CAD build for the part. Positions are in the model's coordinates, mm. Face numbers are marked on the shaded views. Round coordinates to 2 decimals unless told otherwise and drop trailing zeros. Order: outer loops, then holes, each group sorted by start corner. A loop starts at its lowest first (then second) coordinate and runs counter-clockwise, first axis right, second up. Notation, with made-up numbers: (52.5, 54) -> (83.5, 54) arc R17 ccw to (83.5, 66) -> close; hole circle Ø9 at (32, -39). An arc over 180 degrees is marked (long way). Return JSON: item names as keys, results as strings. Group by question number.
Q1. Flat gauge pins, fed straight in: pin 1 (3 mm diameter, centred on y = 1208, z = 845, fed in from +X); pin 2 (3 mm diameter, centred on x = 1200, z = 6, fed in from +Y); pin 3 (5 mm diameter, centred on x = 524.5, z = 487, fed in from -Y). Where does each tip first touch, or does it go through?
Q2. Mould opens along Z. For the marked faces 1, 2 and 3 say: +Z half, -Z half, draft (parallel to the pull), parting line (faces both ways), or undercut.
Q3. Cut at B-B (z = 315). Write the cut outline in (x, y), then the cut area to 3 significant figures.
Q4. Cut at A-A (y = 234). Write the cut outline in (x, z).
Q5. Probe line 1 along Z through (x, y) = (1775, 1221); line 2 along Y through (x, z) = (1104, 408.5); line 3 along X through (y, z) = (845.5, 64). List the from-to ranges inside material, lowest first.
from build123d import *

# Parameters (mm, degrees)
CROQUIS2_W                = 76.2
CROQUIS2_H                = 76.2
SALIENTE_EXTRUIR1_DEPTH   = 900
SALIENTE_EXTRUIR1_2_DEPTH = 900
SALIENTE_EXTRUIR1_3_DEPTH = 900
SALIENTE_EXTRUIR1_4_DEPTH = 900
CROQUIS3_W                = 1852.4
CROQUIS3_H                = 852.4
SALIENTE_EXTRUIR2_DEPTH   = 210
CROQUIS4_W                = 832.4
CROQUIS4_H                = 150
CORTAR_EXTRUIR1_DEPTH     = 1852.4
CROQUIS5_W                = 110
CROQUIS5_H                = 10
SALIENTE_EXTRUIR3_DEPTH   = 220
CROQUIS6_R                = 12.7
SALIENTE_EXTRUIR4_DEPTH   = 40
SALIENTE_EXTRUIR5_START   = -40
CROQUIS7_R                = 12.7
SALIENTE_EXTRUIR5_DEPTH   = 40
CROQUIS8_R                = 44.45
SALIENTE_EXTRUIR6_DEPTH   = 772.4


with BuildPart() as part:
    # Croquis2 → Saliente-Extruir1 (new body)
    with BuildSketch(Plane(origin=(0, 0, 0), x_dir=(1, 0, 0), z_dir=(0, 1, 0))):
        with Locations((38.1, -38.1)):
            Rectangle(CROQUIS2_W, CROQUIS2_H)
    extrude(amount=SALIENTE_EXTRUIR1_DEPTH)



with BuildPart() as body_2:
    # Croquis2 → Saliente-Extruir1 2 (new body)
    with BuildSketch(Plane(origin=(0, 0, 0), x_dir=(1, 0, 0), z_dir=(0, 1, 0))):
        with Locations((1814.3, -38.1)):
            Rectangle(CROQUIS2_W, CROQUIS2_H)
    extrude(amount=SALIENTE_EXTRUIR1_2_DEPTH)


with BuildPart() as body_3:
    # Croquis2 → Saliente-Extruir1 3 (new body)
    with BuildSketch(Plane(origin=(0, 0, 0), x_dir=(1, 0, 0), z_dir=(0, 1, 0))):
        with Locations((1814.3, -814.3)):
            Rectangle(CROQUIS2_W, CROQUIS2_H)
    extrude(amount=SALIENTE_EXTRUIR1_3_DEPTH)


with BuildPart() as body_4:
    # Croquis2 → Saliente-Extruir1 4 (new body)
    with BuildSketch(Plane(origin=(0, 0, 0), x_dir=(1, 0, 0), z_dir=(0, 1, 0))):
        with Locations((38.1, -814.3)):
            Rectangle(CROQUIS2_W, CROQUIS2_H)
    extrude(amount=SALIENTE_EXTRUIR1_4_DEPTH)


with BuildPart() as part_1:
    add(part.part)

    add(body_2.part)  # Saliente-Extruir2 merges body 2

    add(body_3.part)  # Saliente-Extruir2 merges body 3

    add(body_4.part)  # Saliente-Extruir2 merges body 4
    # Croquis3 → Saliente-Extruir2 (add)
    with BuildSketch(Plane(origin=(0, 900, 0), x_dir=(1, 0, 0), z_dir=(0, 1, 0))):
        with Locations((926.2, -426.2)):
            Rectangle(CROQUIS3_W, CROQUIS3_H)
    extrude(amount=SALIENTE_EXTRUIR2_DEPTH)

    # Croquis4 → Cortar-Extruir1 (cut)
    with BuildSketch(Plane.ZY):
        with Locations((426.2, 1035)):
            Rectangle(CROQUIS4_W, CROQUIS4_H)
    extrude(amount=-CORTAR_EXTRUIR1_DEPTH, mode=Mode.SUBTRACT)

    # Croquis5 → Saliente-Extruir3 (add)
    with BuildSketch(Plane(origin=(0, 1110, 0), x_dir=(1, 0, 0), z_dir=(0, 1, 0))):
        with Locations((1747.4, -5)):
            Rectangle(CROQUIS5_W, CROQUIS5_H)
        with Locations((1747.4, -847.4)):
            Rectangle(CROQUIS5_W, CROQUIS5_H)
    extrude(amount=SALIENTE_EXTRUIR3_DEPTH)

    # Croquis6 → Saliente-Extruir4 (add)
    with BuildSketch(Plane.XY.offset(852.4)):
        with Locations((1747.4, 1280)):
            Circle(CROQUIS6_R)
    extrude(amount=-SALIENTE_EXTRUIR4_DEPTH)

    # Croquis7 → Saliente-Extruir5 (add)
    with BuildSketch(Plane(origin=(0, 0, 0), x_dir=(-1, 0, 0), z_dir=(0, 0, -1)).offset(SALIENTE_EXTRUIR5_START)):
        with Locations(Location((-1747.4, 1280, 0), (0, 0, 180))):
            Circle(CROQUIS7_R)
    extrude(amount=SALIENTE_EXTRUIR5_DEPTH)

    # Croquis8 → Saliente-Extruir6 (add)
    with BuildSketch(Plane.XY.offset(40)):
        with Locations((1747.4, 1280)):
            Circle(CROQUIS8_R)
    extrude(amount=SALIENTE_EXTRUIR6_DEPTH)


solid = part_1.part
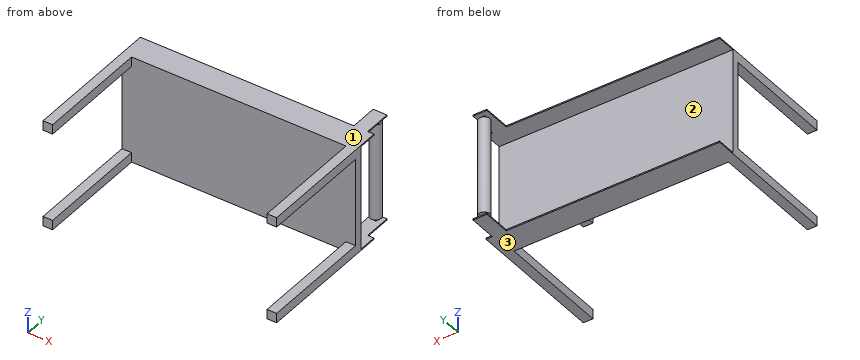
Solution:
{
 "1": {"pin 1": "stops at x = 1802.4", "pin 2": "stops at y = 1110", "pin 3": "stops at y = 900"},
 "2": {"face 1": "+Z half", "face 2": "undercut", "face 3": "-Z half"},
 "3": {"outline": "(0, 900) -> (1852.4, 900) -> (1852.4, 960) -> (0, 960) -> close; circle Ø88.9 at (1747.4, 1280)", "area": "117,000 mm²"},
 "4": {"outline": "(0, 0) -> (76.2, 0) -> (76.2, 76.2) -> (0, 76.2) -> close; (0, 776.2) -> (76.2, 776.2) -> (76.2, 852.4) -> (0, 852.4) -> close; (1776.2, 0) -> (1852.4, 0) -> (1852.4, 76.2) -> (1776.2, 76.2) -> close; (1776.2, 776.2) -> (1852.4, 776.2) -> (1852.4, 852.4) -> (1776.2, 852.4) -> close"},
 "5": {"line 1": "z = 0 to 10, 842.4 to 852.4", "line 2": "y = 900 to 960", "line 3": "x = 0 to 76.2, 1776.2 to 1852.4"}
}
